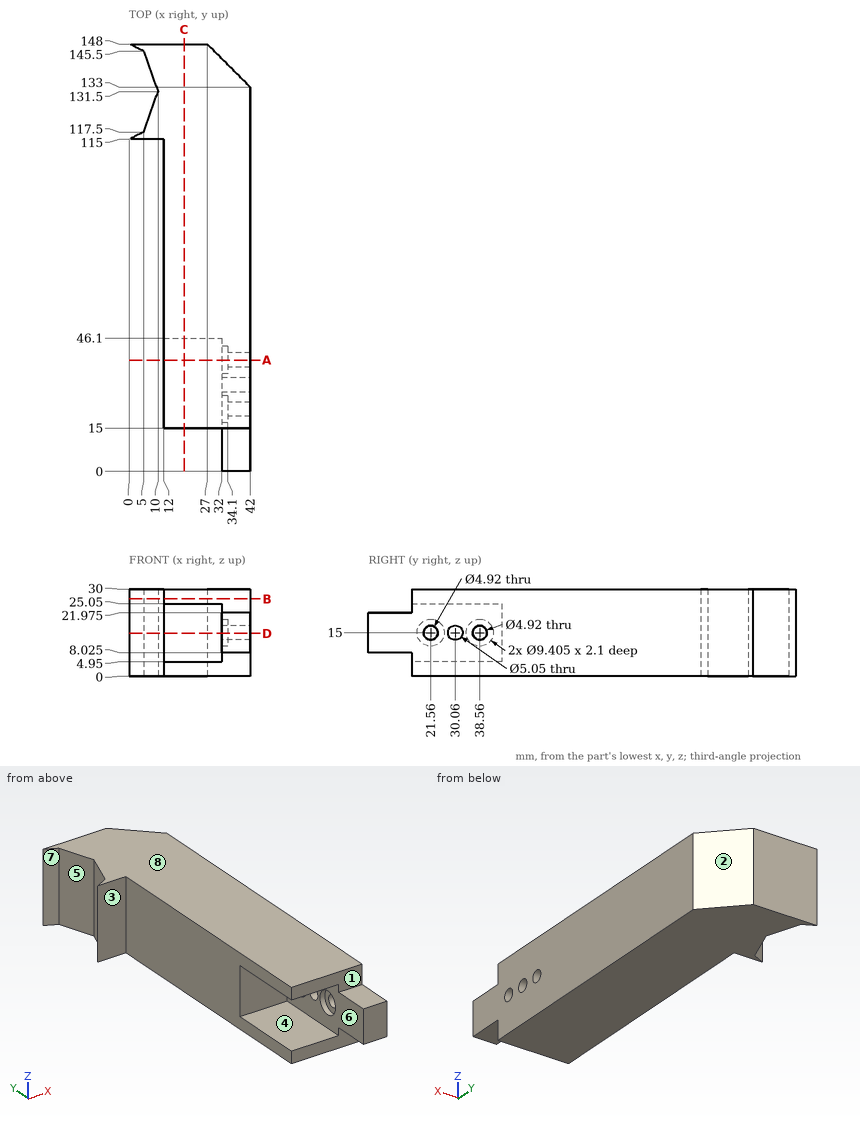
Could you check a few things on this drawing? It's one solid part, dimensions in mm from its lowest x, y, z. A direction names the side the tool comes from. Round coordinates to 2 decimals unless told otherwise and drop trailing zeros. Order: outer loops, then holes, each group sorted by start corner. A loop starts at its lowest first (then second) coordinate and runs counter-clockwise, first axis right, second up.
(1) Imagine slicing it at C-C (x = 19). Write out the boundary of the cut face in (y, z), plus the area to 3 significant figures.
Response values:
outline: (15, 0) - (148, 0) - (148, 30) - (15, 30) - (15, 25.05) - (46.1, 25.05) - (46.1, 4.95) - (15, 4.95) - close
area: 3,360 mm2
(2) Imagine slicing it at D-D (z = 14.75). Count the separate pieces of the cut face and the enclosed holes in it, plus the area to 3 significant figures.
Response values:
separate pieces: 4
enclosed holes: 0
area: 3,410 mm2
(3) Imagine slicing it at A-A (y = 38.56). Write out the boundary of the cut face in (x, z), plus the area to 3 significant figures.
Response values:
outline: (12, 0) - (42, 0) - (42, 12.54) - (34.1, 12.54) - (34.1, 10.3) - (32, 10.3) - (32, 4.95) - (12, 4.95) - close; (12, 25.05) - (32, 25.05) - (32, 19.7) - (34.1, 19.7) - (34.1, 17.46) - (42, 17.46) - (42, 30) - (12, 30) - close
area: 439 mm2
(4) Please list where these lines run through material, in increasing order: line 1 along Z through (x, y) = (36.75, 38.56); line 2 along Y through (x, z) = (33.3, 15) (1 decimal); line 3 along Y through (x, z) = (40, 15) (3 decimals).
Response values:
line 1: z = 0 to 12.54, 17.46 to 30
line 2: y = 0 to 16.9, 26.3 to 27.5, 32.6 to 33.9, 43.3 to 141.7
line 3: y = 0 to 19.1, 24.02 to 27.535, 32.585 to 36.1, 41.02 to 135
(5) Imagine slicing it at B-B (z = 26.75). Write out the boundary of the cut face in (x, y), plus the area to 3 significant figures.
Response values:
outline: (0, 115) - (12, 115) - (12, 15) - (42, 15) - (42, 133) - (27, 148) - (0, 148) - (5, 145.5) - (10, 131.5) - (5, 117.5) - close
area: 4,050 mm2
(6) If we mould it in two halves opening along Z, with no side actions, what happens to the marked faces 6, 7 and 8? For each: released by +Z, released by -Z, zero draft, split by the parting line, or undercut.
Response values:
face 6: undercut
face 7: zero draft
face 8: released by +Z
(7) Which directions (+Z, -Z, +X, -X, +Y, -Y) give clear straight access to the entire face, cutting with the end or side of a thin tool? Please do the marked faces 1, 2, 3, 4 and 5.
Response values:
face 1: +Z, +X, -X, -Y
face 2: +Z, -Z, +X, +Y
face 3: +Z, -Z, -X, -Y
face 4: -X, -Y
face 5: +Z, -Z, -X
(8) I'm going to push flat-ended pins straight in: pin 1 (5 mm diameter, centred on x = 38, y = 9, fed in from +Z) (3 decimals); pin 2 (3 mm diameter, centred on x = 35, z = 22.5, fed in from +Y); pin 3 (4 mm diameter, centred on y = 30.06, z = 15, fed in from +X); pin 4 (6.5 mm diameter, centred on x = 20.5, z = 25.5, fed in from -Y). Where does each tip first touch, or does it pass through?
Response values:
pin 1: stops at z = 21.975
pin 2: stops at y = 141.5
pin 3: passes through
pin 4: stops at y = 15
